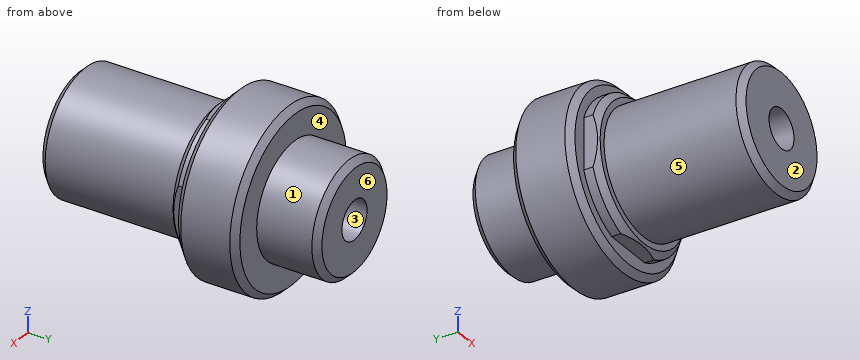
from build123d import *

# Parameters (mm, degrees)
CHAMFER1_SIZE       = 2
SKETCH2_OUTSIDE_W   = 84.354
SKETCH2_OUTSIDE_H   = 84.354
SKETCH2_OUTSIDE_W_2 = 45
SKETCH2_OUTSIDE_H_2 = 45
CUT_EXTRUDE1_DEPTH  = 65.668384857


with BuildPart() as part:
    # Sketch1 → Revolve2 (revolve)
    with BuildSketch(Plane.XY, mode=Mode.PRIVATE) as revolve2_sk:
        Polygon((18.5, 0), (18.5, 20), (6.35, 20), (6.35, -70), (20, -70), (20, -25), (24, -25), (24, -20), (29, -20), (29, 0), align=None)
    revolve(revolve2_sk.sketch.rotate(Axis((0, 38.250415552, 0), (0, -1, 0)), 90), axis=Axis((0, 38.250415552, 0), (0, -1, 0)))

    # Chamfer1
    chamfer1_edges = [part.edges().sort_by_distance(p)[0] for p in [
        (0, -20, -29),
        (0, 0, -29),
        (0, 20, -18.5),
        (0, -70, -20),
        (0, -25, -24),
    ]]
    chamfer(chamfer1_edges, length=CHAMFER1_SIZE)

    # Sketch2 outside → Cut-Extrude1 (cut, through all)
    with BuildSketch(Plane.XZ.offset(20)):
        Rectangle(SKETCH2_OUTSIDE_W, SKETCH2_OUTSIDE_H)
        Rectangle(SKETCH2_OUTSIDE_W_2, SKETCH2_OUTSIDE_H_2, mode=Mode.SUBTRACT)
    extrude(amount=CUT_EXTRUDE1_DEPTH, mode=Mode.SUBTRACT)


solid = part.part
For this review, take the finished solid that the model builds, in its own axes (mm). Face numbers are marked on the shaded views. A direction names the side the tool comes from. Give positions to 0.01 mm unless a question says otherwise; leave off trailing zeros. Loops run counter-clockwise (first coordinate to the right, second up) from the corner with the lowest first, then second, coordinate; pieces in that order, holes last. Notation, with made-up numbers: M 1,68.5 L 26,68.5 A21 cw 26,96.5 Z; hole C -27,60.5 d9. An arc over 180 degrees is marked long. Answer as a JSON object with one key per item and string values. Group by question number.
Q1. For probe 1 along X at (y, z) = (-48, 0); probe 2 along Y at (x, z) = (-3, -26); probe 3 along Z at (x, y) = (-3, -29), list the stretches that pass through material, from the lowest coordinate up. Write a range as [from, to].
Q2. Insertion check: P1, Ø1.5, axis at x = 19.5, z = -0.5, coming from the -Y side; P2, Ø5, axis at x = 5.5, y = -9, coming from the -Z side; P3, Ø1.5, axis at y = -16.5, z = -17.5, coming from the -X side. Each pin has a flat end and moves straight along its axis. Give the tip position at first contact, or say it passes through.
Q3. Add section C-C on y = -29.5. Give the boundary of the cut face in (x, z), and give its area (3 significant figures).
Q4. Mouldability with a two-part tool opening along Z and no side actions: class the marked faces 1, 2 and 3 as +Z half, -Z half, draft (parallel to the pull), parting line (faces both ways), or undercut.
Q5. Add section D-D on y = 12. Give the boundary of the cut face in (x, z).
Q6. Tool access review of the marked faces 4, 5 and 6: name each direction out of +Z, -Z, +X, -X, +Y, -Y from which nothing blocks a thin tool from reaching the whole face with its end or side.
Checked values:
{
 "1": {"probe 1": "[-20, -6.35], [6.35, 20]", "probe 2": "[-20, 0]", "probe 3": "[-19.77, -5.6], [5.6, 19.77]"},
 "2": {"P1": "y = -69.24", "P2": "z = -28.84", "P3": "x = -23.67"},
 "3": {"outline": "C 0,0 d40; hole C 0,0 d12.7", "area": "1,130 mm²"},
 "4": {"face 1": "parting line", "face 2": "draft", "face 3": "undercut"},
 "5": {"outline": "C 0,0 d37; hole C 0,0 d12.7"},
 "6": {"face 4": "+Y", "face 5": "-Y", "face 6": "+Z, -Z, +X, -X, +Y"}
}
